Source: CAD feature listing. Evaluate the final solid. Frame: model axes, mm. Face numbers are marked on the shaded views. A direction names the side the tool comes from. Give positions to 0.01 mm unless a question says otherwise; leave off trailing zeros. Order: outer loops, then holes, each group sorted by start corner. A loop starts at its lowest first (then second) coordinate and runs counter-clockwise, first axis right, second up. Notation, with made-up numbers: M -31,46 L -23,46 A30 ccw -23,74 Z; hole C 70.5,34 d6. An arc over 180 degrees is marked long. Answer in a Markdown table with one row per item. Add a question column.
(1) Mould query, pull axis Y, two halves, no side actions, for the marked faces 1, 2 and 3. Classes: pulls with the +Y half, pulls with the -Y half, needs draft (parallel to the pull), parting line crosses it, or undercut.
(2) Section query A-A, the plane y = 4.75. Return loops of the section in (x, z), plus the area to 3 significant figures.
(3) Section query C-C, the plane z = 1. Return loops of the section in (x, y).
(4) Pin query (flat end, axial travel): P1, Ø3, axis at y = 0, z = 4, coming from the -X side. Return the tip coordinate at first contact, or that it passes through.
(5) Set-up query: the marked faces 4 and 5. Return all of +Z, -Z, +X, -X, +Y, -Y with unobstructed straight access to the full face (end or side cutting, diameter ignored); none if empty.
(6) Section query B-B, the plane x = -48. Return loops of the section in (y, z), plus the area to 4 significant figures.
(7) Section query D-D, the plane y = 0. Return loops of the section in (x, z).
(8) Material intervals for line 1 along Y through (x, z) = (-16.5, 2.5); line 2 along X through (y, z) = (-6.25, 1.5); line 3 along Y through (x, z) = (-55.8, 4), sorted ascending.
Autodesk Inventor part; units mm, degrees
ref_plane "YZ Plane" through (0, 0, 0) normal (1, 0, 0) x (0, 1, 0)
ref_plane "XZ Plane" through (0, 0, 0) normal (0, 1, 0) x (-1, 0, 0)
ref_plane "XY Plane" through (0, 0, 0) normal (0, 0, 1) x (1, 0, 0)
sketch "Sketch2" plane through (0, 0, 0) normal (0, 0, 1) x (1, 0, 0)
  line L0 (-54, 11.5) -> (54, 11.5)
  line L1 (55, 10.5) -> (55, -10.5)
  line L2 (54, -11.5) -> (-54, -11.5)
  line L3 (-55, -10.5) -> (-55, 10.5)
  line L4 (-55, 11.5) -> (55, -11.5) construction
  line L5 (55, 11.5) -> (-55, -11.5) construction
  line L6 (53, 9.5) -> (-53, 9.5)
  line L7 (-53, 9.5) -> (-53, -9.5)
  line L8 (-53, -9.5) -> (53, -9.5)
  line L9 (53, -9.5) -> (53, 9.5)
  line L10 (57, 13.5) -> (-57, 13.5)
  line L11 (-57, 13.5) -> (-57, -13.5)
  line L12 (-57, -13.5) -> (57, -13.5)
  line L13 (57, -13.5) -> (57, 13.5)
  arc A0 (55, 10.5) -> (54, 11.5) centre (54, 10.5) ccw
  arc A1 (54, -11.5) -> (55, -10.5) centre (54, -10.5) ccw
  arc A2 (-55, -10.5) -> (-54, -11.5) centre (-54, -10.5) ccw
  arc A3 (-54, 11.5) -> (-55, 10.5) centre (-54, 10.5) ccw
  point P0 (0, 0)
  dimension "d0" = 110
  dimension "d1" = 23
  dimension "d2" = 2
  dimension "d3" = 2
  dimension "d10" = 1
extrude "Extrusion2" add sketch "Sketch2" along normal blind 12 contours L13 L12 L11 L10
sketch "Sketch3" plane through (-57, -13.5, 0) normal (-1, 0, 0) x (0, 0, 1)
  line L0 (7, 19.5) -> (9, 19.5)
  line L1 (9, 19.5) -> (9, 7.5)
  line L2 (9, 7.5) -> (7, 7.5)
  line L3 (7, 7.5) -> (7, 19.5)
  line L4 (0, 27) -> (0, 0)
  line L5 (0, 27) -> (12, 27)
  circle A0 centre (4, 13.5) radius 2
  line L6 (12, 27) -> (12, 0)
  line L7 (0, 13.5) -> (2, 13.5) construction
  line L8 (12, 0) -> (12, 27) construction
  line L9 (0, 0) -> (0, 27) construction
  dimension "d20" = 4
  dimension "d12" = 2
  dimension "d13" = 12
  dimension "d15" = 7.5
  dimension "d21" = 3
  dimension "d24" = 4
  dimension "d25" = 2
  dimension "d26" = 3
extrude "Extrusion4" cut sketch "Sketch3" against normal blind 10
extrude "Extrusion5" add sketch "Sketch2" against normal blind 2 contours L0 A0 L1 A1 L2 A2 L3 A3 | L9 L8 L7 L6 | L13 L12 L11 L10
sketch "Sketch4" plane through (-54, 11.5, 12) normal (0, -1, 0) x (1, 0, 0)
  line L0 (3.4899, -1) -> (43.4899, -1)
  line L1 (43.4899, -1) -> (43.4899, 0)
  line L2 (43.4899, 0) -> (3.4899, 0)
  line L3 (3.4899, 0) -> (3.4899, -1)
  line L4 (0, 0) -> (108, 0)
  point P0 (54, -12)
  dimension "d27" = 1
  dimension "d28" = 40
extrude "Extrusion6" cut sketch "Sketch4" against normal blind 0.5
properties part number "sdm_finger_bone_attachment_mould"
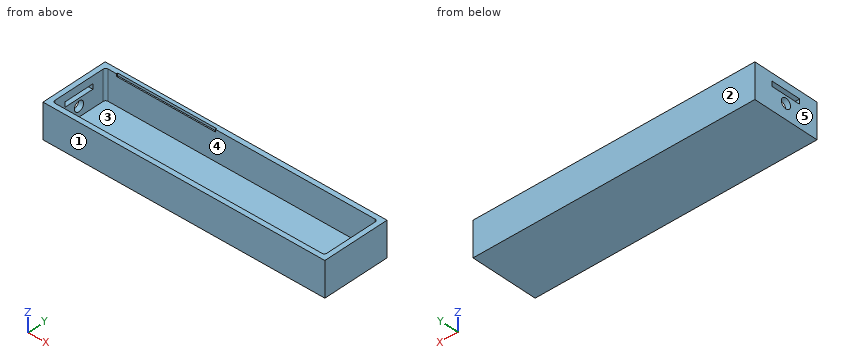
Values follow:
| question | item | result |
|---|---|---|
| 1 | face 1 | pulls with the -Y half |
| 1 | face 2 | pulls with the +Y half |
| 1 | face 3 | undercut |
| 2 | outline | M -57,-2 L 57,-2 L 57,12 L 55,12 L 55,0 L -55,0 L -55,7 L -57,7 Z; M -57,9 L -55,9 L -55,12 L -57,12 Z |
| 2 | area | 272 mm² |
| 3 | outline | M -57,-13.5 L 57,-13.5 L 57,13.5 L -57,13.5 Z; hole M -55,-10.5 A1 ccw -54,-11.5 L 54,-11.5 A1 ccw 55,-10.5 L 55,10.5 A1 ccw 54,11.5 L -54,11.5 A1 ccw -55,10.5 Z |
| 4 | P1 | stops at x = 55 |
| 5 | face 4 | +Z |
| 5 | face 5 | +Z, -Z, -X, +Y, -Y |
| 6 | outline | M -13.5,-2 L 13.5,-2 L 13.5,12 L 12,12 L 12,11 L 11.5,11 L 11.5,0 L -11.5,0 L -11.5,12 L -13.5,12 Z |
| 6 | area | 101.5 mm² |
| 7 | outline | M -57,-2 L 57,-2 L 57,12 L 55,12 L 55,0 L -55,0 L -55,2 L -57,2 Z; M -57,6 L -55,6 L -55,7 L -57,7 Z; M -57,9 L -55,9 L -55,12 L -57,12 Z |
| 8 | line 1 | y = -13.5 to -11.5, 11.5 to 13.5 |
| 8 | line 2 | x = -57 to -55, 55 to 57 |
| 8 | line 3 | y = -13.5 to -2, 2 to 13.5 |
